Study the drawing (mm; zero at the part's minimum x, y, z) and answer. A direction names the side the tool comes from. Give positions to 0.01 mm unless a question says otherwise; leave off trailing zeros. Write each loop counter-clockwise with the first axis right and the second up, starting at its lowest first coordinate (ties: lowest second). Pieces come first, ordered by that corner, then holes. Notation, with made-up numbers: (27.5, 21) -> (63.5, 21) arc R15 cw to (63.5, 48) -> close; hole circle Ø3 at (47, 19.5). An arc over 180 degrees is marked (long way). One line per question, with ' | ' between items.
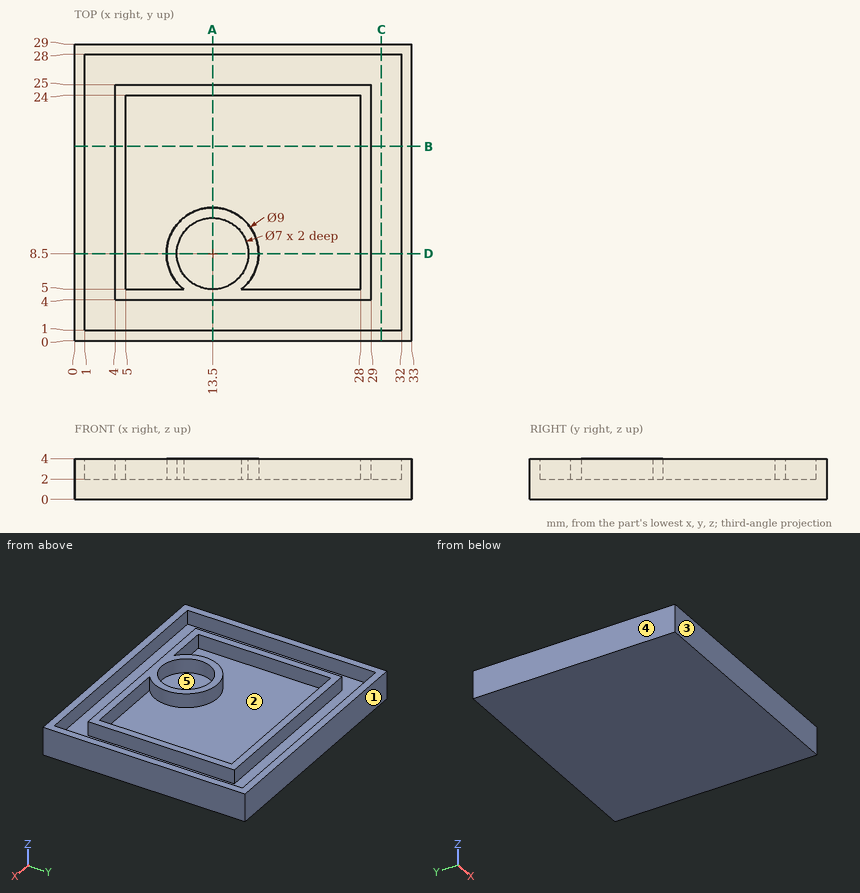
Item 1: Flat-ended cylindrical pins translate along their axes: pin 1 (1.6 mm diameter, centred on x = 16, z = 3.5, fed in from -Y); pin 2 (4 mm diameter, centred on x = 13.5, y = 8.5, fed in from +Z). Find the tip coordinate at first contact, or state that the pin passes through.
Answers below:
pin 1: y = 0 | pin 2: z = 2
Item 2: Find section A-A (x = 13.5). Write down the section's boundary in (y, z), then the cut area to 3 significant figures.
Answers below:
outline: (0, 0) -> (29, 0) -> (29, 4) -> (28, 4) -> (28, 2) -> (25, 2) -> (25, 4) -> (24, 4) -> (24, 2) -> (13, 2) -> (13, 4) -> (12, 4) -> (12, 2) -> (5, 2) -> (5, 4) -> (4, 4) -> (4, 2) -> (1, 2) -> (1, 4) -> (0, 4) -> close | area: 68.0 mm²
Item 3: Find section D-D (y = 8.5). Write down the section's boundary in (x, z).
Answers below:
outline: (0, 0) -> (33, 0) -> (33, 4) -> (32, 4) -> (32, 2) -> (29, 2) -> (29, 4) -> (28, 4) -> (28, 2) -> (18, 2) -> (18, 4) -> (17, 4) -> (17, 2) -> (10, 2) -> (10, 4) -> (9, 4) -> (9, 2) -> (5, 2) -> (5, 4) -> (4, 4) -> (4, 2) -> (1, 2) -> (1, 4) -> (0, 4) -> close
Item 4: Find section B-B (y = 19). Write down the section's boundary in (x, z).
Answers below:
outline: (0, 0) -> (33, 0) -> (33, 4) -> (32, 4) -> (32, 2) -> (29, 2) -> (29, 4) -> (28, 4) -> (28, 2) -> (5, 2) -> (5, 4) -> (4, 4) -> (4, 2) -> (1, 2) -> (1, 4) -> (0, 4) -> close
Item 5: Consider line 1 (Y direction, x = 13.5, z = 2.55); line 2 (X direction, y = 8.5, z = 2.7); line 3 (Y direction, x = 8, z = 2.4). Determine where each line is inside the solid, lowest interval first. Write a range as [from, to].
Answers below:
line 1: [0, 1], [4, 5], [12, 13], [24, 25], [28, 29] | line 2: [0, 1], [4, 5], [9, 10], [17, 18], [28, 29], [32, 33] | line 3: [0, 1], [4, 5], [24, 25], [28, 29]
Item 6: A tool of negligible diameter and unlimited length cuts with its end or side. For the marked faces 1 and 2, from which of +Z, -Z, +X, -X, +Y, -Y can it reach the whole face along a straight path? Write none if from no direction.
Answers below:
face 1: +Z, -Z, +X, -X, +Y | face 2: +Z
Item 7: Determine the mould class of the marked faces 3, 4 and 5 for opening direction X: pulls with the +X half, pulls with the -X half, needs draft (parallel to the pull), parting line crosses it, or undercut.
Answers below:
face 3: needs draft | face 4: pulls with the -X half | face 5: undercut
Item 8: Find section C-C (x = 30). Write down the section's boundary in (y, z), then the cut area to 3 significant figures.
Answers below:
outline: (0, 0) -> (29, 0) -> (29, 4) -> (28, 4) -> (28, 2) -> (1, 2) -> (1, 4) -> (0, 4) -> close | area: 62.0 mm²
